The model under review builds one solid part; all positions refer to its coordinate system, in mm. Round coordinates to 2 decimals unless told otherwise and drop trailing zeros. Loops run counter-clockwise (first coordinate to the right, second up) from the corner with the lowest first, then second, coordinate; pieces in that order, holes last. Notation, with made-up numbers: (-18.75, 8) -> (20.25, 8) arc R27 cw to (20.25, 26) -> close; hole circle Ø7 at (-12.5, 68.5). An arc over 180 degrees is marked (long way). Return JSON: item names as keys, results as strings. Group by question number.
Autodesk Inventor part; units mm, degrees
ref_plane "YZ Plane" through (0, 0, 0) normal (1, 0, 0) x (0, 1, 0)
ref_plane "XZ Plane" through (0, 0, 0) normal (0, 1, 0) x (-1, 0, 0)
ref_plane "XY Plane" through (0, 0, 0) normal (0, 0, 1) x (1, 0, 0)
sketch "Esquisse1" plane through (0, 0, 0) normal (0, 0, 1) x (1, 0, 0)
  circle A0 centre (0, 0) radius 6
  line L0 (-3.3166, 5) -> (3.3166, 5)
  line L1 (-3.3166, -5) -> (3.3166, -5)
  dimension "d0" = 12
  dimension "d1" = 10
  dimension "d2" = 5
extrude "Extrusion1" add sketch "Esquisse1" along normal blind 1 contours A0 L1 L0
fillet "Congé1" radius 0.5 4 edges at (-3.3166, 5, 0.5) (3.3166, 5, 0.5) (-3.3166, -5, 0.5) (3.3166, -5, 0.5)
sketch "Esquisse2" plane through (0, 0, 1) normal (0, 0, 1) x (1, 0, 0)
  arc A0 (-3.4498, 4.9091) -> (-3.4498, -4.9091) centre (0, 0) ccw
  circle A1 centre (0, 0) radius 2.5
  dimension "d6" = 5
extrude "Extrusion2" add sketch "Esquisse2" along normal blind 1
fillet "Congé2" radius 0.3 1 edges at (-2.5, 0, 2)
properties part number "plaque moteur" material "Résine acétal, noir"
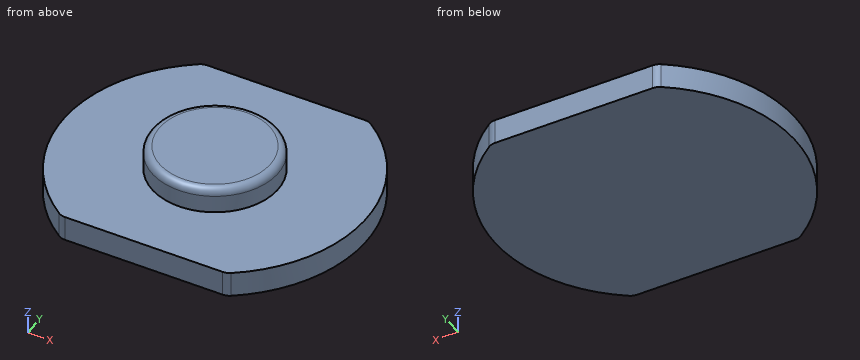
1. We need section B-B, the plane x = 0. Write out the cut boundary in (y, z).
2. We need section D-D, the plane z = 1.4. Write out the cut boundary in (x, y), then the cut area to 3 significant figures.
3. We need section C-C, the plane y = 0. Write out the cut boundary in (x, z), then the cut area to 3 significant figures.
4. We need section A-A, the plane z = 0.3. Write out the cut boundary in (x, y), then the cut area to 3 significant figures.
5. Wall thickness on line 1 (Z direction, x = 3.5, y = 4.5); line 2 (X direction, y = -3.5, z = 0.65); line 3 (X direction, y = -0.25, z = 0.15): over which ranges is each line inside the solid? List them lowest first.
6. For P1, Ø1, axis at x = 4, y = 3, coming from the +Z side, flat-tipped, find the tip position at first contact; note if it passes through.
Check sheet entries:
{
 "1": {"outline": "(-5, 0) -> (5, 0) -> (5, 1) -> (2.5, 1) -> (2.5, 1.7) arc R0.3 ccw to (2.2, 2) -> (-2.2, 2) arc R0.3 ccw to (-2.5, 1.7) -> (-2.5, 1) -> (-5, 1) -> close"},
 "2": {"outline": "circle Ø5 at (0, 0)", "area": "19.6 mm²"},
 "3": {"outline": "(-6, 0) -> (6, 0) -> (6, 1) -> (2.5, 1) -> (2.5, 1.7) arc R0.3 ccw to (2.2, 2) -> (-2.2, 2) arc R0.3 ccw to (-2.5, 1.7) -> (-2.5, 1) -> (-6, 1) -> close", "area": "17.0 mm²"},
 "4": {"outline": "(-3.45, -4.91) arc R0.5 ccw to (-3.16, -5) -> (3.16, -5) arc R0.5 ccw to (3.45, -4.91) arc R6 ccw to (3.45, 4.91) arc R0.5 ccw to (3.16, 5) -> (-3.16, 5) arc R0.5 ccw to (-3.45, 4.91) arc R6 ccw to start", "area": "104 mm²"},
 "5": {"line 1": "z = 0 to 1", "line 2": "x = -4.87 to 4.87", "line 3": "x = -5.99 to 5.99"},
 "6": {"P1": "stops at z = 1"}
}
